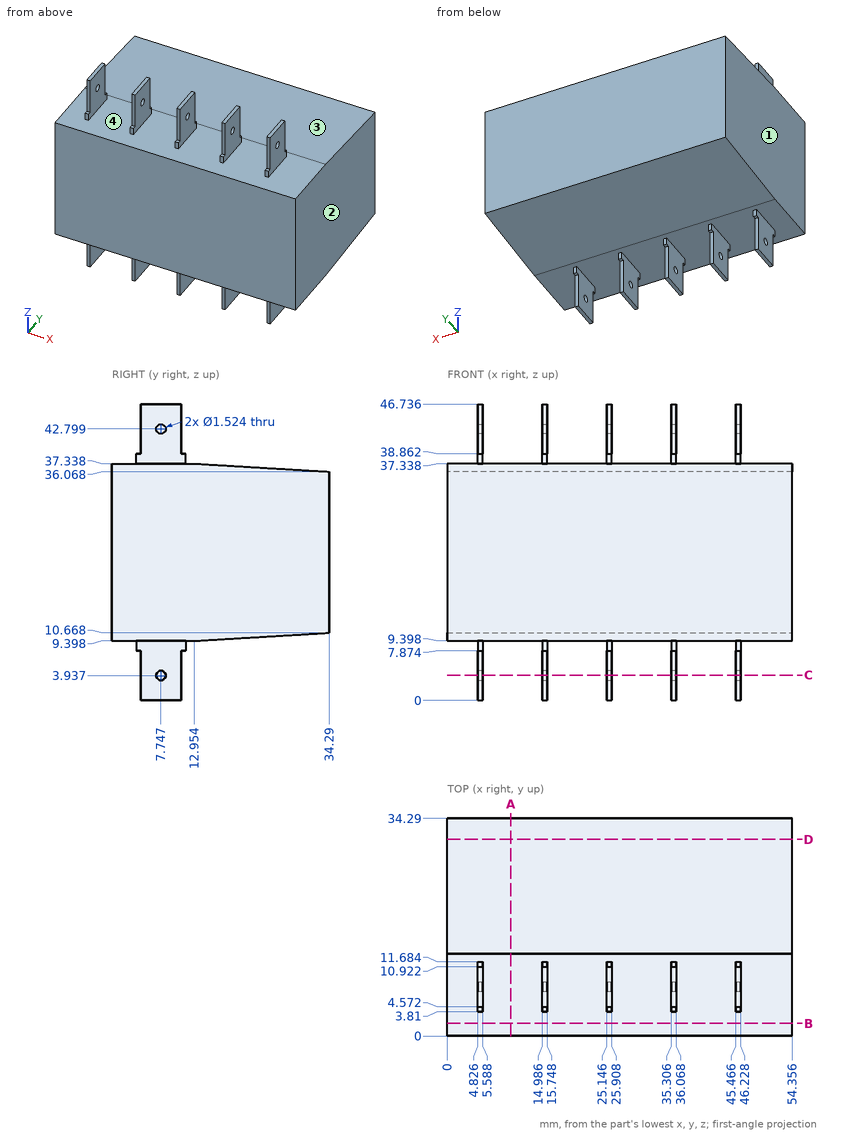
Input: dimensioned drawing with shaded views. Units: mm. Origin: part minimum x, y, z. Give positions to 0.01 mm unless a question says otherwise; leave off trailing zeros. Write each loop counter-clockwise with the first axis right and the second up, starting at its lowest first coordinate (ties: lowest second). Pieces come first, ordered by that corner, then holes.
1. Section query B-B (y = 2). Return the cut outline in (x, z), then the cut area to 3 significant figures.
2. Material intervals for line 1 along Z through (x, y) = (23.5, 6.5); line 2 along Z through (x, y) = (48, 32.5), sorted ascending.
3. Section query D-D (y = 31). Return the cut outline in (x, z), then the cut area to 3 significant figures.
4. Pull-direction query (X, two-part tool) for the marked faces 1, 2, 3 and 4; classes: +X half, -X half, draft (parallel to the pull), parting line (faces both ways), or undercut.
5. First-contact query: pin 1 (8 mm diameter, centred on x = 21.5, y = 27.5, fed in from +Z); pin 2 (0.6 mm diameter, centred on x = 45.5, z = 44, fed in from -Y); pin 3 (5 mm diameter, centred on x = 30.5, y = 30.5, fed in from +Z). Flat tips, straight axial feed; report the tip coordinate or a pass-through.
6. Section query A-A (x = 10). Return the cut outline in (y, z), then the cut area to 3 significant figures.
7. Section query C-C (z = 4). Count the separate pieces of the cut face and the enclosed holes in it, then the cut area to 3 significant figures.
Output values:
1. outline: (0, 9.4) - (54.36, 9.4) - (54.36, 37.34) - (0, 37.34) - close
1. area: 1,520 mm2
2. line 1: z = 9.4 to 37.34
2. line 2: z = 10.56 to 36.17
3. outline: (0, 10.47) - (54.36, 10.47) - (54.36, 36.26) - (0, 36.26) - close
3. area: 1,400 mm2
4. face 1: -X half
4. face 2: +X half
4. face 3: draft
4. face 4: undercut
5. pin 1: stops at z = 36.71
5. pin 2: stops at y = 4.57
5. pin 3: stops at z = 36.44
6. outline: (0, 9.4) - (12.95, 9.4) - (34.29, 10.67) - (34.29, 36.07) - (12.95, 37.34) - (0, 37.34) - close
6. area: 931 mm2
7. separate pieces: 10
7. enclosed holes: 0
7. area: 18.4 mm2
